```python
from build123d import *

# Parameters (mm, degrees)
F0_W     = 2.304975711
F0_H     = 7.7243503183
F0_W_2   = 3.6289574255
F0_H_2   = 6.098523736
F0_H_3   = 5.3181350231
F0_H_4   = 0.6922000066
F1_DEPTH = 12.7


with BuildPart() as f1:
    # F0 (on Top) → F1 (new body)
    with BuildSketch(Plane.XY):
        with BuildLine():
            Line((-34.5030121262, 0), (-37.2290474303, 0))
            Line((-37.2290474303, 0), (-37.2290474303, -3.256221069))
            Line((-37.2290474303, -3.256221069), (37.2290474303, -3.256221069))
            Line((37.2290474303, -3.256221069), (37.2290474303, 0))
            Line((37.2290474303, 0), (35.4276069029, 0))
            Line((35.4276069029, 0), (35.0221842527, 0))
            Line((35.0221842527, 0), (32.7145940604, 0))
            Line((32.7145940604, 0), (23.4078748053, 0))
            Line((23.4078748053, 0), (21.1028990943, 0))
            Line((21.1028990943, 0), (14.9383603664, 0))
            add(Edge.make_bspline(
                [(14.9383603664, 0), (13.4825928521, -0.2734716945), (11.6876593256, -0.2734716945)],
                knots=[0.406741787, 0.406741787, 0.406741787, 1, 1, 1], degree=2))
            add(Edge.make_bspline(
                [(11.6876593256, -0.2734716945), (10.2835431713, -0.2734716945), (9.0848653779, 0)],
                knots=[0, 0, 0, 0.3205826669, 0.3205826669, 0.3205826669], degree=2))
            Line((9.0848653779, 0), (0.8486304171, 0))
            Line((0.8486304171, 0), (-1.5388208843, 0))
            Line((-1.5388208843, 0), (-14.3963313476, 0))
            Line((-14.3963313476, 0), (-16.7316928024, 0))
            Line((-16.7316928024, 0), (-19.444705645, 0))
            Line((-19.444705645, 0), (-21.749681356, 0))
            Line((-21.749681356, 0), (-32.1980364151, 0))
            Line((-32.1980364151, 0), (-34.5030121262, 0))
        make_face()
        Polygon((-34.5030121262, 19.833209084), (-34.5030121262, 0), (-32.1980364151, 0), (-32.1980364151, 9.3327641783), (-21.749681356, 9.3327641783), (-21.749681356, 0), (-19.444705645, 0), (-19.444705645, 19.833209084), (-21.749681356, 19.833209084), (-21.749681356, 11.3946539386), (-32.1980364151, 11.3946539386), (-32.1980364151, 19.833209084), align=None)
        Polygon((35.0221842527, 0), (35.4276069029, 0), (35.0221842527, 0.5496391018), align=None)
        Polygon((-8.8921708927, 19.9156846744), (-16.7316928024, 0), (-14.3963313476, 0), (-11.9567901996, 6.3072122563), (-4.0087477761, 6.3072122563), (-1.5388208843, 0), (0.8486304171, 0), (-6.9518241077, 19.9156846744), align=None)
        with BuildLine():
            Line((-7.0342996981, 14.5287263743), (-4.7249831665, 8.3821244783))
            Line((-4.7249831665, 8.3821244783), (-11.1407159366, 8.3821244783))
            Line((-11.1407159366, 8.3821244783), (-8.8096953023, 14.5287263743))
            add(Edge.make_bspline(
                [(-7.9545536543, 17.3893271155), (-8.2540702721, 16.0870809511), (-8.8096953023, 14.5287263743)],
                knots=[0, 0, 0, 1, 1, 1], degree=2))
            add(Edge.make_bspline(
                [(-7.0342996981, 14.5287263743), (-7.4814042146, 15.6964071017), (-7.9545536543, 17.3893271155)],
                knots=[0, 0, 0, 1, 1, 1], degree=2))
        make_face(mode=Mode.SUBTRACT)
        Polygon((32.7145940604, 0), (35.0221842527, 0), (35.0221842527, 0.5496391018), (27.1540029383, 11.2166802962), (35.0221842527, 19.7187706114), (35.0221842527, 19.833209084), (32.4020549809, 19.833209084), (26.9062852626, 13.8228740543), (27.0378924906, 13.8228740543), (27.0378924906, 7.7243503183), (26.9108741687, 7.7243503183), align=None)
        Polygon((27.1540029383, 11.2166802962), (35.0221842527, 0.5496391018), (35.0221842527, 19.7187706114), align=None)
        Polygon((35.0221842527, 19.833209084), (35.0221842527, 19.7187706114), (35.1280902851, 19.833209084), align=None)
        with Locations((22.2553869498, 3.8621751592)):
            Rectangle(F0_W, F0_H)
        Polygon((25.4871278479, 9.6192583345), (26.9108741687, 7.7243503183), (27.0378924906, 7.7243503183), (27.0378924906, 13.8228740543), (26.9062852626, 13.8228740543), (23.4078748053, 9.9969097222), (23.4078748053, 13.8228740543), (21.1028990943, 13.8228740543), (21.1028990943, 7.7243503183), (23.4078748053, 7.7243503183), (23.4078748053, 7.7744096016), align=None)
        with BuildLine():
            add(Edge.make_bspline(
                [(9.0848653779, 0), (6.544483275, 0.579574096), (4.926831322, 2.3874513014)],
                knots=[0.3205826669, 0.3205826669, 0.3205826669, 1, 1, 1], degree=2))
            Line((9.0848653779, 0), (14.9383603664, 0))
            add(Edge.make_bspline(
                [(16.7751010079, 0.5035351836), (15.9364442822, 0.1874940174), (14.9383603664, 0)],
                knots=[0, 0, 0, 0.406741787, 0.406741787, 0.406741787], degree=2))
            Line((16.7751010079, 0.5035351836), (16.7751010079, 2.5220167384))
            add(Edge.make_bspline(
                [(12.03926579, 1.7753956042), (14.114178012, 1.7753956042), (16.7751010079, 2.5220167384)],
                knots=[0, 0, 0, 1, 1, 1], degree=2))
            add(Edge.make_bspline(
                [(6.8367923632, 3.9002272624), (8.6621074036, 1.7753956042), (12.03926579, 1.7753956042)],
                knots=[0, 0, 0, 1, 1, 1], degree=2))
            add(Edge.make_bspline(
                [(5.0114773227, 9.9144341317), (5.0114773227, 6.0250589207), (6.8367923632, 3.9002272624)],
                knots=[0, 0, 0, 1, 1, 1], degree=2))
            add(Edge.make_bspline(
                [(6.9040750817, 15.8765511545), (5.0114773227, 13.6996296496), (5.0114773227, 9.9144341317)],
                knots=[0, 0, 0, 1, 1, 1], degree=2))
            add(Edge.make_bspline(
                [(12.0653107133, 18.0534726593), (8.7966728406, 18.0534726593), (6.9040750817, 15.8765511545)],
                knots=[0, 0, 0, 1, 1, 1], degree=2))
            add(Edge.make_bspline(
                [(16.5710824422, 16.9986532662), (14.3181965777, 18.0534726593), (12.0653107133, 18.0534726593)],
                knots=[0, 0, 0, 1, 1, 1], degree=2))
            Line((16.5710824422, 16.9986532662), (17.5477670655, 18.9780674361))
            add(Edge.make_bspline(
                [(12.0956964571, 20.1153624196), (15.2124056106, 20.1153624196), (17.5477670655, 18.9780674361)],
                knots=[0, 0, 0, 1, 1, 1], degree=2))
            add(Edge.make_bspline(
                [(7.001743544, 18.8673765121), (9.1656425872, 20.1153624196), (12.0956964571, 20.1153624196)],
                knots=[0, 0, 0, 1, 1, 1], degree=2))
            add(Edge.make_bspline(
                [(3.6918678761, 15.3144148935), (4.8378445008, 17.6193906045), (7.001743544, 18.8673765121)],
                knots=[0, 0, 0, 1, 1, 1], degree=2))
            add(Edge.make_bspline(
                [(2.5458912514, 9.9448198756), (2.5458912514, 13.0094391825), (3.6918678761, 15.3144148935)],
                knots=[0, 0, 0, 1, 1, 1], degree=2))
            add(Edge.make_bspline(
                [(4.926831322, 2.3874513014), (2.5458912514, 5.0483742974), (2.5458912514, 9.9448198756)],
                knots=[0, 0, 0, 1, 1, 1], degree=2))
        make_face()
        with BuildLine():
            Line((14.9383603664, 0), (9.0848653779, 0))
            add(Edge.make_bspline(
                [(11.6876593256, -0.2734716945), (10.2835431713, -0.2734716945), (9.0848653779, 0)],
                knots=[0, 0, 0, 0.3205826669, 0.3205826669, 0.3205826669], degree=2))
            add(Edge.make_bspline(
                [(14.9383603664, 0), (13.4825928521, -0.2734716945), (11.6876593256, -0.2734716945)],
                knots=[0.406741787, 0.406741787, 0.406741787, 1, 1, 1], degree=2))
        make_face()
        with Locations((19.2884203816, 10.7736121863)):
            Rectangle(F0_W_2, F0_H_2)
        Polygon((23.4078748053, 9.9969097222), (26.9062852626, 13.8228740543), (23.4078748053, 13.8228740543), align=None)
        with Locations((22.2553869498, 16.4819415659)):
            Rectangle(F0_W, F0_H_3)
        with Locations((22.2553869498, 19.4871090807)):
            Rectangle(F0_W, F0_H_4)
        Polygon((21.039057523, 19.1410090774), (21.1028990943, 19.1410090774), (21.1028990943, 19.833209084), (23.4078748053, 19.833209084), (23.4078748053, 19.1410090774), (23.4089195728, 19.1410090774), (23.4089195728, 48.1270328164), (21.039057523, 48.1270328164), align=None)
    extrude(amount=F1_DEPTH)


solid = f1.part
```
The model under review builds one solid part; all positions refer to its coordinate system, in mm. A direction names the side the tool comes from. Give positions to 0.01 mm unless a question says otherwise; leave off trailing zeros. Write each loop counter-clockwise with the first axis right and the second up, starting at its lowest first coordinate (ties: lowest second). Pieces come first, ordered by that corner, then holes. Notation, with made-up numbers: M -18,52 L -13,52 A23 cw -13,90 Z; hole C 34,79.25 d11. An arc over 180 degrees is marked long. Write each question's results on one line, items separated by ' | '. Start each with the question number.
1. Insertion check: pin 1 Ø7 at (y, z) = (16, 3.5) entering from -X; pin 2 Ø7 at (x, z) = (17, 6.5) entering from +Y; pin 3 Ø0.9 at (x, z) = (36.5, 4) entering from +Y; pin 4 Ø2 at (x, y) = (-16, 9.5) entering from -Z (3 decimals). Each pin has a flat end and moves straight along its axis. Give the tip position at first contact, or say it passes through.
2. We need section C-C (z = 11.25). Count the separate pieces of the cut face and the enclosed holes in it, and give its area (3 significant figures).
3. For probe 1 along X at (y, z) = (19, 8.5); probe 2 along Y at (x, z) = (-29.5, 9.5); probe 3 along Y at (x, z) = (19, 3.25), list the stretches that pass through material, from the lowest coordinate up. Write a range as [from, to].
4. We need section A-A (x = 31). Write out the cut boundary in (y, z), and give its area (3 significant figures).
5. For faces 1 (the flat face through (34, 19.833, 6)), 2 (the flat face through (-13.194, 3.109, 6.261)), 3 (the flat face through (-27, 11.395, 6)), list the 3-axis set-ups (+Z, -Z, +X, -X, +Y, -Y) from which the entire face can be reached by the end or side of a thin tool; tool diameter is ignored.
6. Mouldability with a two-part tool opening along X and no side actions: class faces 4 (the flat face through (37.229, -2, 6)), 5 (the flat face through (-8, 0, 6)), 6 (the flat face through (-32.198, 5, 6)), 7 (the flat face through (-34.503, 10, 6)) as released by +X, released by -X, zero draft, split by the parting line, or undercut.
7. We need section B-B (y = 25.5). Write out the cut boundary in (x, z), and give its area (3 significant figures).
Results found:
1) pin 1: stops at x = -34.5 | pin 2: stops at y = 20.05 | pin 3: stops at y = 0 | pin 4: passes through
2) separate pieces: 1 | enclosed holes: 4 | area: 817 mm^2
3) probe 1: x = [-34.5, -32.2], [-21.75, -19.44], [-9.25, -6.59], [7.24, 17.5], [21.1, 23.41], [31.64, 35.02] | probe 2: y = [-3.26, 0], [9.33, 11.39] | probe 3: y = [-3.26, 0], [7.72, 13.82]
4) outline: M -3.26,0 L 0,0 L 0,12.7 L -3.26,12.7 Z; M 2.28,0 L 18.3,0 L 18.3,12.7 L 2.28,12.7 Z | area: 245 mm^2
5) face 1: +Z, -Z, +X, +Y | face 2: +Z, -Z | face 3: +Z, -Z, +Y
6) face 4: released by +X | face 5: undercut | face 6: undercut | face 7: released by -X
7) outline: M 21.04,0 L 23.41,0 L 23.41,12.7 L 21.04,12.7 Z | area: 30.1 mm^2
